```python
from build123d import *

# Parameters (mm, degrees)
F1_DEPTH = 125.222
F2_R     = 2.25
F3_DEPTH = 1.525
F4_R     = 1.7526
F5_DEPTH = 25.4


with BuildPart() as f1:
    # F0 (on Front) → F1 (new body)
    with BuildSketch(Plane.XZ):
        with BuildLine():
            Line((0, 1.524), (0, 0))
            Line((0, 0), (9.652, 0))
            ThreePointArc((9.652, 0), (11.807261, 0.892739), (12.7, 3.048))
            ThreePointArc((12.7, 3.048), (13.146369, 4.125631), (14.224, 4.572))
            Line((14.224, 4.572), (181.864, 4.572))
            ThreePointArc((181.864, 4.572), (182.941631, 4.125631), (183.388, 3.048))
            ThreePointArc((183.388, 3.048), (184.280739, 0.892739), (186.436, 0))
            Line((186.436, 0), (196.088, 0))
            Line((196.088, 0), (196.088, 1.524))
            Line((196.088, 1.524), (186.436, 1.524))
            ThreePointArc((186.436, 1.524), (185.358369, 1.970369), (184.912, 3.048))
            ThreePointArc((184.912, 3.048), (184.019261, 5.203261), (181.864, 6.096))
            Line((181.864, 6.096), (14.224, 6.096))
            ThreePointArc((14.224, 6.096), (12.068739, 5.203261), (11.176, 3.048))
            ThreePointArc((11.176, 3.048), (10.729631, 1.970369), (9.652, 1.524))
            Line((9.652, 1.524), (0, 1.524))
        make_face()
    extrude(amount=F1_DEPTH)

    # F2 (on face) → F3 (cut, through all)
    with BuildSketch(Plane.XY.offset(1.524)):
        with Locations((5.08, -112.649)):
            Circle(F2_R)
        with Locations((191.008, -112.649)):
            Circle(F2_R)
        with Locations((191.008, -12.573)):
            Circle(F2_R)
        with Locations((5.08, -12.573)):
            Circle(F2_R)
    extrude(amount=-F3_DEPTH, mode=Mode.SUBTRACT)

    # F4 (on face) → F5 (cut)
    with BuildSketch(Plane.XY.offset(6.096)):
        with Locations((16.002, -12.573)):
            Circle(F4_R)
        with Locations((16.002, -42.545)):
            Circle(F4_R)
        with Locations((16.002, -112.649)):
            Circle(F4_R)
        with Locations((180.086, -112.649)):
            Circle(F4_R)
        with Locations((180.086, -42.545)):
            Circle(F4_R)
        with Locations((180.086, -12.573)):
            Circle(F4_R)
    extrude(amount=-F5_DEPTH, mode=Mode.SUBTRACT)


solid = f1.part
```
The model under review builds one solid part; all positions refer to its coordinate system, in mm. A direction names the side the tool comes from. Round coordinates to 2 decimals unless told otherwise and drop trailing zeros. Loops run counter-clockwise (first coordinate to the right, second up) from the corner with the lowest first, then second, coordinate; pieces in that order, holes last. Notation, with made-up numbers: (-28, 55) - (18, 55) arc R19 ccw to (18, 92) - close; hole circle Ø1 at (34, 15.25). An arc over 180 degrees is marked (long way). Write each question's results on one line, items separated by ' | '. Start each with the question number.
Q1. Take a section at A-A on x = 5.08. Give the boundary of the cut face in (y, z).
Q2. Tool access review of faces 4 (the flat face through (97, -62, 4.572)), 5 (the flat face through (191, -62, 1.524)), 6 (the flat face through (5, -62, 0)), 7 (the flat face through (5, -62, 1.524)): name each direction out of +Z, -Z, +X, -X, +Y, -Y from which nothing blocks a thin tool from reaching the whole face with its end or side.
Q3. Take a section at C-C on x = 154.5. Give the boundary of the cut face in (y, z), plus the area to 3 significant figures.
Q4. Take a section at B-B on y = -24.5. Give the boundary of the cut face in (x, z).
Q5. Wall thickness on line 1 along X through (y, z) = (-117, 3); line 2 along Y through (x, z) = (5.08, 0.5); line 3 along Z through (x, y) = (123, -33.5): over which ranges is each line inside the solid? List them lowest first. Write a range as [from, to].
Q6. Insertion check: P1, Ø10.5, axis at x = 4.5, y = -73, coming from the +Z side; P2, Ø1, axis at x = 76, y = -33.5, coming from the -Z side; P3, Ø1.5, axis at y = -58.5, z = 2.5, coming from the +X side. Each pin has a flat end and moves straight along its axis. Give the tip position at first contact, or say it passes through.
Q7. Draft analysis for pull direction X (two halves, no side actions). For faces 1 (the cylindrical face through (193.1, -13.4, 0.8)), 2 (the cylindrical face through (15.774, -40.807, 5.345)), 3 (the flat face through (99, -62, 6.096)), state which applies: pulls with the +X half, pulls with the -X half, needs draft (parallel to the pull), parting line crosses it, or undercut.
Data:
1) outline: (-125.22, 0) - (-114.9, 0) - (-114.9, 1.52) - (-125.22, 1.52) - close; (-110.4, 0) - (-14.82, 0) - (-14.82, 1.52) - (-110.4, 1.52) - close; (-10.32, 0) - (0, 0) - (0, 1.52) - (-10.32, 1.52) - close
2) face 4: -Z, +Y, -Y | face 5: +Z, +X, +Y, -Y | face 6: -Z, +X, -X, +Y, -Y | face 7: +Z, -X, +Y, -Y
3) outline: (-125.22, 4.57) - (0, 4.57) - (0, 6.1) - (-125.22, 6.1) - close | area: 191 mm²
4) outline: (0, 0) - (9.65, 0) arc R3.05 ccw to (12.7, 3.05) arc R1.52 cw to (14.22, 4.57) - (181.86, 4.57) arc R1.52 cw to (183.39, 3.05) arc R3.05 ccw to (186.44, 0) - (196.09, 0) - (196.09, 1.52) - (186.44, 1.52) arc R1.52 cw to (184.91, 3.05) arc R3.05 ccw to (181.86, 6.1) - (14.22, 6.1) arc R3.05 ccw to (11.18, 3.05) arc R1.52 cw to (9.65, 1.52) - (0, 1.52) - close
5) line 1: x = [11.18, 12.7], [183.39, 184.91] | line 2: y = [-125.22, -114.9], [-110.4, -14.82], [-10.32, 0] | line 3: z = [4.57, 6.1]
6) P1: stops at z = 1.53 | P2: stops at z = 4.57 | P3: stops at x = 185.64
7) face 1: undercut | face 2: undercut | face 3: needs draft
